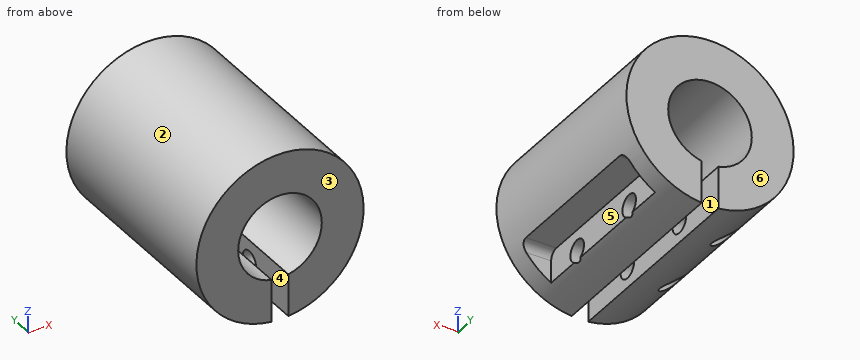
Autodesk Inventor part; units mm, degrees
ref_plane "Arbeitsebene1" through (20, 0, 0) normal (1, 0, 0) x (0, 0, -1)
ref_plane "YZ Plane" through (0, 0, 0) normal (1, 0, 0) x (0, 1, 0)
ref_plane "XZ Plane" through (0, 0, 0) normal (0, 1, 0) x (-1, 0, 0)
sketch "Skizze1" plane through (0, 0, 0) normal (0, 1, 0) x (-1, 0, 0)
  circle A0 centre (0, 0) radius 10
  circle A1 centre (0, 0) radius 20
  dimension "d0" = 20
  dimension "d1" = 40
extrude "Extrusion1" add sketch "Skizze1" along normal blind 50
sketch "Skizze2" plane through (0, 50, 0) normal (0, 1, 0) x (1, 0, 0)
  line L0 (0, 0) -> (2, 0)
  line L1 (2, 0) -> (2, 25)
  line L2 (2, 25) -> (0, 25)
  line L3 (0, 25) -> (0, 0)
  line L4 (0, 0) -> (-2, 0)
  line L5 (-2, 0) -> (-2, 25)
  line L6 (-2, 25) -> (0, 25)
  line L7 (0, 25) -> (0, 0)
  dimension "d4" = 2
  dimension "d5" = 25
  dimension "d6" = 2
  dimension "d7" = 25
extrude "Extrusion2" cut sketch "Skizze2" against normal blind 50
ref_plane "Arbeitsebene1" through (20, 0, 0) normal (1, 0, 0) x (0, 0, -1)
sketch "Skizze5" plane through (20, 0, 0) normal (1, 0, 0) x (0, 0, -1)
  line L0 (0, 0) -> (10, 0)
  line L1 (-10, 0) -> (9.798, 0)
  line L2 (10, 0) -> (10, 5)
  line L3 (10, 7) -> (10, 43)
  line L4 (12, 45) -> (18, 45)
  line L5 (20, 43) -> (20, 7)
  line L6 (18, 5) -> (12, 5)
  arc A0 (18, 5) -> (20, 7) centre (18, 7) ccw
  arc A1 (10, 7) -> (12, 5) centre (12, 7) ccw
  arc A2 (12, 45) -> (10, 43) centre (12, 43) ccw
  arc A3 (20, 43) -> (18, 45) centre (18, 43) ccw
  point P0 (10, 45)
  point P1 (20, 45)
  dimension "d11" = 10
  dimension "d12" = 5
  dimension "d13" = 40
  dimension "d14" = 10
  dimension "d15" = 2
extrude "Extrusion3" cut sketch "Skizze5" against normal blind 10
sketch "Skizze6" plane through (20, 0, 0) normal (1, 0, 0) x (0, 0, -1)
  line L0 (17.3205, 5) -> (12, 5)
  line L1 (15, 5) -> (15, 15)
  line L2 (15, 15) -> (15, 35)
  circle A0 centre (15, 15) radius 2.5
  circle A1 centre (15, 35) radius 2.5
  point P0 (0, 0)
  point P1 (18, 5)
  dimension "d18" = 10
  dimension "d19" = 20
  dimension "d20" = 5
  dimension "d21" = 5
extrude "Extrusion4" cut sketch "Skizze6" against normal through all
thread "Gewinde1"
sketch "Skizze8" plane through (20, 0, 0) normal (1, 0, 0) x (0, 0, -1)
  circle A0 centre (15, 35) radius 2.5
  circle A1 centre (15, 35) radius 2.6
  arc A2 (17.3205, 15.9302) -> (17.3205, 14.0698) centre (15, 15) ccw
  circle A3 centre (15, 15) radius 2.6
  point P0 (0, 0)
  point P1 (14.8661, 37.4964)
  point P2 (14.8661, 32.5036)
  dimension "d30" = 5.2
  dimension "d31" = 5.2
extrude "Extrusion6" cut sketch "Skizze8" against normal blind 25 contours A0 | A1 | A3
thread "Gewinde2"
thread "Gewinde3"
equation "\"d0\" = durchmesser"
properties part number "StoperKlein" material "PVC, hart"
The listing builds one solid part. Answer for the finished solid, in the listing's coordinates (mm). Face numbers are marked on the shaded views. A direction names the side the tool comes from. Coordinates: 2 decimals unless noted, no trailing zeros. Write each loop counter-clockwise with the first axis right and the second up, starting at its lowest first coordinate (ties: lowest second). Pieces come first, ordered by that corner, then holes. Notation, with made-up numbers: M 71,-5 L 102,-5 A19 ccw 102,4 Z; hole C -15,-19.75 d3. An arc over 180 degrees is marked long. Put each result on its own line as item: value. Start each with the question number.
1. A cutting plane is placed at A-A on z = 0. Write down the section's boundary in (x, y), then the cut area to 3 significant figures.
2. Flat-ended cylindrical pins translate along their axes: P1, Ø8.5, axis at y = 35, z = -15, coming from the -X side; P2, Ø1, axis at y = 11, z = 6.5, coming from the +X side; P3, Ø3.5, axis at x = 14.5, y = 27, coming from the -Z side. Find the tip coordinate at first contact, or state that the pin passes through.
3. A cutting plane is placed at D-D on y = 15. Write down the section's boundary in (x, z).
4. Which of the six approach directions +Z, -Z, +X, -X, +Y, -Y give full straight-line access (tool end or side, diameter ignored) to the marked faces 5 and 6?
5. A cutting plane is placed at B-B on x = 5. Write down the section's boundary in (y, z).
6. Consider line 1 (Y direction, x = 8.25, z = -15); line 2 (Y direction, x = -9.5, z = -15); line 3 (Z direction, x = -9, y = 15). Determine where each line is inside the solid, lowest interval first. Write a range as from..to.
7. A cutting plane is placed at C-C on y = 26. Write down the section's boundary in (x, z), then the cut area to 3 significant figures.
8. For a pull along X with two mould halves and no side action, classify the marked faces 1, 2, 3 and 4 as pulls with the +X half, pulls with the -X half, needs draft (parallel to the pull), parting line crosses it, or undercut.
Resolved:
1. outline: M -20,0 L -10,0 L -10,50 L -20,50 Z; M 10,0 L 20,0 L 20,50 L 10,50 Z
1. area: 1,000 mm2
2. P1: stops at x = -16.87
2. P2: stops at x = 19.08
2. P3: stops at z = -10
3. outline: M -15.61,-12.5 L -5,-12.5 L -5,-12.4 L -2,-12.4 L -2,-9.8 A10 cw long 2,-9.8 L 2,-12.4 L 10,-12.4 L 10,-10 L 17.32,-10 A20 ccw long Z; M -9.68,-17.5 A20 ccw -2,-19.9 L -2,-17.6 L -5,-17.6 L -5,-17.5 Z; M 2,-19.9 A20 ccw 9.5,-17.6 L 2,-17.6 Z
4. face 5: -Z, +X
4. face 6: +Z, -Z, +X, -X, +Y
5. outline: M 0,-19.36 L 50,-19.36 L 50,-8.66 L 0,-8.66 Z; M 0,8.66 L 50,8.66 L 50,19.36 L 0,19.36 Z; hole C 15,-15 d5.2; hole C 35,-15 d5.2
6. line 1: y = 0..12.4, 17.6..32.4, 37.6..50
6. line 2: y = 0..12.5, 17.5..32.5, 37.5..50
6. line 3: z = -17.86..-17.5, -12.5..-4.36, 4.36..17.86
7. outline: M -2,-19.9 L -2,-9.8 A10 cw long 2,-9.8 L 2,-19.9 A20 ccw 10,-17.32 L 10,-10 L 17.32,-10 A20 ccw long Z
7. area: 871 mm2
8. face 1: undercut
8. face 2: parting line crosses it
8. face 3: needs draft
8. face 4: undercut
